The listing builds one solid part. Answer for the finished solid, in the listing's coordinates (mm). Face numbers are marked on the shaded views. A direction names the side the tool comes from. Coordinates: 2 decimals unless noted, no trailing zeros. Return JSON: item names as keys, results as strings. Group by question number.
1. Straight lines are drawn through the part: L1, parallel to Y at x = 17, z = 8; L2, parallel to X at y = -26, z = 45; L3, parallel to Y at x = 25, z = -26.5 (3 decimals). For each, find the intervals that lie inside material, in ascending order. Write a range as from..to.
2. Given P1, Ø8.5, axis at x = 17, y = 29.14, coming from the -Z side; P2, Ø10, axis at x = -24, z = -12, coming from the +Y side; P3, Ø1, axis at x = 18.5, z = 28.5, coming from the +Y side, each flat-ended and moving along its own axis, determine where each tip first touches the part or whether it passes through.
3. Which of the six approach directions +Z, -Z, +X, -X, +Y, -Y give full straight-line access (tool end or side, diameter ignored) to the marked faces 1, 2, 3 and 4?
4. The mould has two halves that part along X. Classify the marked faces 5, 6 and 7: pulls with the +X half, pulls with the -X half, needs draft (parallel to the pull), parting line crosses it, or undercut.
5. Section A-A (y = 0) is taken. Count the separate pieces of the cut face and the enclosed holes in it, then the cut area to 3 significant figures.
```python
from build123d import *

# Parameters (mm, degrees)
BOSS_EXTRUDE1_DEPTH      = 37
BOSS_EXTRUDE1_DEPTH_BACK = 52
CUT_EXTRUDE5_REACH       = 108.479
SKETCH11_R               = 6.4
SKETCH12_R               = 6.4
CUT_EXTRUDE6_DEPTH       = 107.479320653
SKETCH14_R               = 12.9
CUT_EXTRUDE8_DEPTH       = 96.517571793
SKETCH15_R               = 12.9
CUT_EXTRUDE9_DEPTH       = 96.055320399
SKETCH16_R               = 2.625
CUT_EXTRUDE10_DEPTH      = 128.687117596
SKETCH13_R               = 6.4
CUT_EXTRUDE15_DEPTH      = 103.003266712
CUT_EXTRUDE16_DEPTH      = 128.687117596
CUT_EXTRUDE17_DEPTH      = 125.149710579
CUT_EXTRUDE25_DEPTH      = 117.949180331
SKETCH31_R               = 2.625
CUT_EXTRUDE22_DEPTH      = 103.253619099
CUT_EXTRUDE26_DEPTH      = 125.149710659
SKETCH36_R               = 2.625
CUT_EXTRUDE27_DEPTH      = 95.867859136


with BuildPart() as part:
    # Sketch9 → Boss-Extrude1 (new, two sides: drawn at the far end of the back side and taken through both)
    with BuildSketch(Plane(origin=(0, 0, 0), x_dir=(1, 0, 0), z_dir=(0, 1, 0)).offset(-BOSS_EXTRUDE1_DEPTH_BACK)):
        Polygon((-5, 50), (5, 50), (10, 37.5), (40, 37.5), (40, -37.5), (10, -37.5), (5, -50), (-5, -50), (-60, -50), (-60, 50), align=None)
    extrude(amount=BOSS_EXTRUDE1_DEPTH + BOSS_EXTRUDE1_DEPTH_BACK)

    # Cut-Extrude5: up to this plane
    cut_extrude5_end = Plane(origin=(40, -52, 37.5), z_dir=(1, 0, 0))
    # Sketch11 → Cut-Extrude5 (cut, up to the surface)
    with BuildSketch(Plane(origin=(12.990381057, 0, -7.5), x_dir=(-0.5000000000000013, 0, -0.8660254037844379), z_dir=(0.8660254037844379, 0, -0.5000000000000013)), mode=Mode.PRIVATE) as cut_extrude5_sk1:
        with Locations(Location((0, 0, 0), (0, 0, 180))):
            Circle(SKETCH11_R)
    cut_extrude5_tool1 = split(extrude(cut_extrude5_sk1.sketch, amount=CUT_EXTRUDE5_REACH, mode=Mode.PRIVATE), bisect_by=cut_extrude5_end, keep=Keep.BOTH, mode=Mode.PRIVATE)
    add(cut_extrude5_tool1.solids().sort_by_distance((12.990381, 0, -7.5))[0], mode=Mode.SUBTRACT)

    # Sketch12 → Cut-Extrude6 (cut, through all)
    with BuildSketch(Plane(origin=(12.990381057, 0, 7.5), x_dir=(0.5000000000000009, 0, -0.866025403784438), z_dir=(0.8660254037844382, 0, 0.500000000000001))):
        Circle(SKETCH12_R)
    extrude(amount=CUT_EXTRUDE6_DEPTH, mode=Mode.SUBTRACT)

    # Sketch14 → Cut-Extrude8 (cut, through all)
    with BuildSketch(Plane(origin=(-3.229283171, -7.476383099, -12.59664344), x_dir=(-0.9697475532809772, 0.007782671596180618, 0.24398588674016475), z_dir=(-0.21528554474375752, -0.49842553993010197, -0.8397762293431328))):
        with Locations(Location((0, 0, 0), (0, 0, 116.704243504))):
            Circle(SKETCH14_R)
    extrude(amount=CUT_EXTRUDE8_DEPTH, mode=Mode.SUBTRACT)

    # Sketch15 → Cut-Extrude9 (cut, through all)
    with BuildSketch(Plane(origin=(-3.798019855, -7.5, 12.422763186), x_dir=(-0.9674136083951571, 0.13086508264944213, -0.2167607908156276), z_dir=(0.2532013236376571, 0.49999999999999495, -0.8281842124238686))):
        with Locations(Location((0, 0, 0), (0, 0, 90))):
            Circle(SKETCH15_R)
    extrude(amount=-CUT_EXTRUDE9_DEPTH, mode=Mode.SUBTRACT)

    # Sketch16 → Cut-Extrude10 (cut, through all)
    with BuildSketch(Plane(origin=(0, 0, -50), x_dir=(-1, 0, 0), z_dir=(0, 0, -1))):
        with Locations((-25, 0)):
            Circle(SKETCH16_R)
    extrude(amount=-CUT_EXTRUDE10_DEPTH, mode=Mode.SUBTRACT)

    # Sketch13 → Cut-Extrude15 (cut, through all)
    with BuildSketch(Plane(origin=(5, 8.660254038, 0), x_dir=(0.8581606322585569, -0.49545927204241474, -0.1344635228929922), z_dir=(0.49999999999999806, 0.8660254037844397, 0))):
        with Locations(Location((0, 0, 0), (0, 0, 172.272400829))):
            Circle(SKETCH13_R)
    extrude(amount=CUT_EXTRUDE15_DEPTH, mode=Mode.SUBTRACT)

    # Sketch25 → Cut-Extrude16 (cut, through all)
    with BuildSketch(Plane.XY.offset(50)):
        Polygon((-60, -65.770666842), (-0.665327834, 37), (-60, 37), align=None)
    extrude(amount=-CUT_EXTRUDE16_DEPTH, mode=Mode.SUBTRACT)

    # Sketch26 → Cut-Extrude17 (cut, through all)
    with BuildSketch(Plane(origin=(0, 0, -50), x_dir=(-1, 0, 0), z_dir=(0, 0, -1))):
        Polygon((-40, -14), (-17.898055975, -19.831365478), (0.674513826, -52), (-40, -52), align=None)
    extrude(amount=-CUT_EXTRUDE17_DEPTH, mode=Mode.SUBTRACT)

    # Sketch27 → Cut-Extrude25 (cut, through all)
    with BuildSketch(Plane.ZY.offset(-40)):
        Polygon((-50, 37), (-15.598651273, 37), (-15.598651273, 25), (-50, 5.138372052), align=None)
        Polygon((15.537544719, 37), (15.537544719, 25), (50, 5.103092167), (50, 37), align=None)
    extrude(amount=CUT_EXTRUDE25_DEPTH, mode=Mode.SUBTRACT)

    # Sketch31 → Cut-Extrude22 (cut, through all)
    with BuildSketch(Plane(origin=(22.010775129, -12.707926946, 0), x_dir=(0, 0, -1), z_dir=(0.8660254037844397, -0.4999999999999981, 0))):
        with Locations(Location((-27.712190923, -18.725438309, 0), (0, 0, 90))):
            Circle(SKETCH31_R)
        with Locations(Location((29.158933157, -18.725438309, 0), (0, 0, 90))):
            Circle(SKETCH31_R)
    extrude(amount=-CUT_EXTRUDE22_DEPTH, mode=Mode.SUBTRACT)

    # Sketch35 → Cut-Extrude26 (cut, through all)
    with BuildSketch(Plane(origin=(0, 0, -50), x_dir=(-1, 0, 0), z_dir=(0, 0, -1))):
        Polygon((44.639977993, -39.16632832), (25.461488573, -60.033808877), (52.049501792, -52), align=None)
    extrude(amount=-CUT_EXTRUDE26_DEPTH, mode=Mode.SUBTRACT)

    # Sketch36 → Cut-Extrude27 (cut, through all)
    with BuildSketch(Plane(origin=(0, 0, -15.598651273), x_dir=(-1, 0, 0), z_dir=(0, 0, -1))):
        with Locations((-17, 29.136428333)):
            Circle(SKETCH36_R)
    extrude(amount=-CUT_EXTRUDE27_DEPTH, mode=Mode.SUBTRACT)


solid = part.part
```
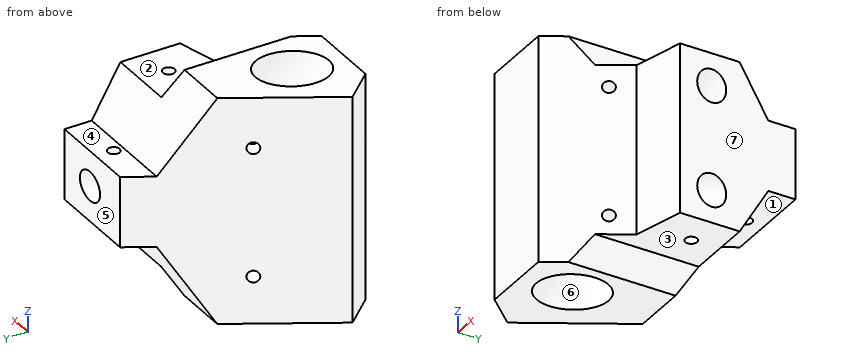
Worked out:
{
 "1": {"L1": "-21.39..-6.2, 6.2..26.51, 31.76..37", "L2": "-37.04..-26.89, -0.31..7", "L3": "-17.958..-2.625, 2.625..18.706"},
 "2": {"P1": "z = -15.79", "P2": "y = 5.24", "P3": "y = 17.8"},
 "3": {"face 1": "-Z, +X, -X, +Y", "face 2": "+Z, +X, +Y, -Y", "face 3": "-Z, +X, +Y, -Y", "face 4": "+Z, +X, -X, +Y"},
 "4": {"face 5": "needs draft", "face 6": "undercut", "face 7": "pulls with the +X half"},
 "5": {"separate pieces": "4", "enclosed holes": "2", "area": "4,130 mm^2"}
}
